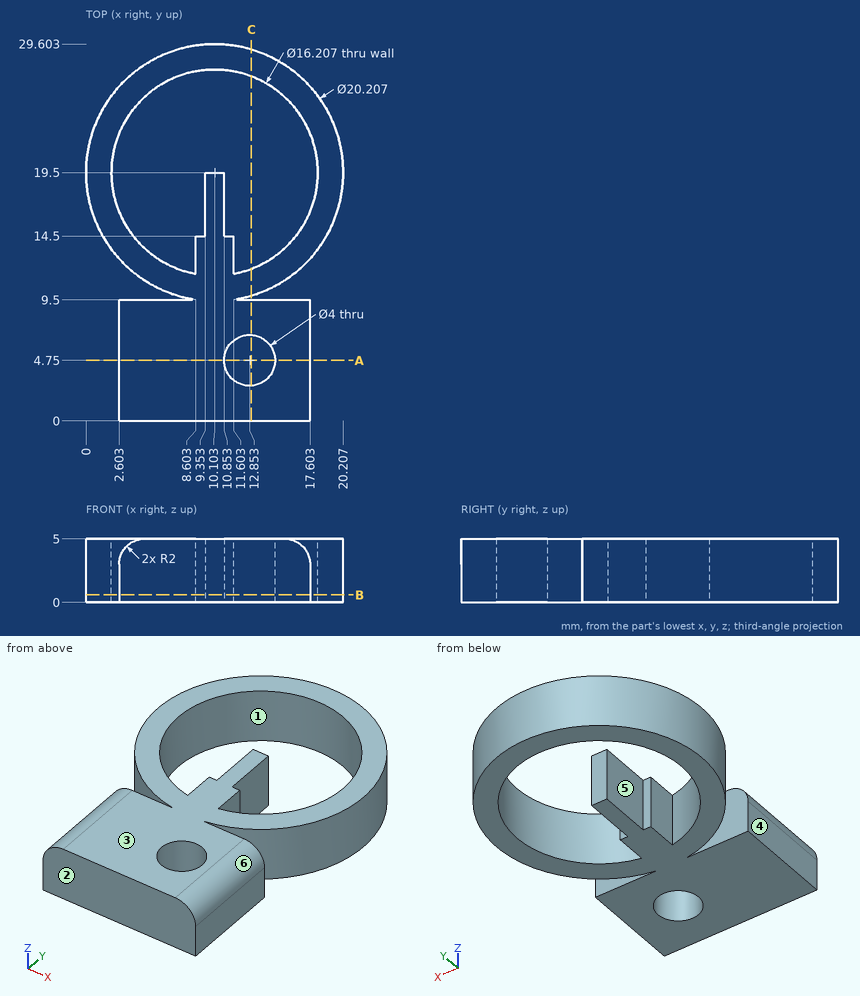
Input: dimensioned drawing with shaded views. Units: mm. Origin: part minimum x, y, z. A direction names the side the tool comes from. Round coordinates to 2 decimals unless told otherwise and drop trailing zeros. Order: outer loops, then holes, each group sorted by start corner. A loop starts at its lowest first (then second) coordinate and runs counter-clockwise, first axis right, second up. Notation, with made-up numbers: M 10,-8.75 L 65,-8.75 A32 cw 65,26.25 Z; hole C 6,7.5 d6. An arc over 180 degrees is marked long. Use one line per item in the form item = value. Start each with the question number.
Q1. Cut plane C-C (x = 13). Return loops of the section in (y, z) (1 decimal).
Q2. Cut plane A-A (y = 4.75). Return loops of the section in (x, z).
Q3. Access query for the marked faces 4, 5 and 6. Directions: +Z, -Z, +X, -X, +Y, -Y. A direction counts if a zero-diameter tool reaches every point of the face in a straight line with its end or side. Return the directions, or none.
Q4. Cut plane B-B (z = 0.6). Count the separate pieces of the cut face and the enclosed holes in it, and give its area (3 significant figures).
Q5. Mould query, pull axis Y, two halves, no side actions, for the marked faces 1, 2 and 3. Classes: +Y half, -Y half, draft (parallel to the pull), parting line (faces both ways), or undercut.
Q6. Pin query (flat end, axial travel): pin 1 Ø0.9 at (y, z) = (4.5, 1) entering from +X; pin 2 Ø2 at (x, z) = (3.5, 1.5) entering from +Y; pin 3 Ø2.5 at (x, z) = (14.5, 3) entering from +Y. Return the tip coordinate at first contact, or that it passes through.
Q7. Material intervals for line 1 (X direction, y = 19.25, z = 0.65); line 2 (Y direction, x = 16.75, z = 4.1) (1 decimal); line 3 (X direction, y = 18, z = 4.6) (1 decimal), sorted ascending. Write a range as [from, to].
Geometry results:
q1.outline = M 0,0 L 2.8,0 L 2.8,5 L 0,5 Z; M 6.7,0 L 9.5,0 L 9.5,5 L 6.7,5 Z; M 9.8,0 L 11.9,0 L 11.9,5 L 9.8,5 Z; M 27.1,0 L 29.2,0 L 29.2,5 L 27.1,5 Z
q2.outline = M 2.6,0 L 10.85,0 L 10.85,5 L 4.6,5 A2 ccw 2.6,3 Z; M 14.85,0 L 17.6,0 L 17.6,3 A2 ccw 15.6,5 L 14.85,5 Z
q3.face_4 = +Z, -Z, -X, -Y
q3.face_5 = +Z, -Z
q3.face_6 = +Z, +X, -Y
q4.separate_pieces = 1
q4.enclosed_holes = 2
q4.area = 261 mm^2
q5.face_1 = undercut
q5.face_2 = -Y half
q5.face_3 = draft
q6.pin_1 = 17.6
q6.pin_2 = 27.91
q6.pin_3 = 29.1
q7.line_1 = [0, 2], [9.35, 10.85], [18.2, 20.2]
q7.line_2 = [0, 9.5], [11.9, 14.9], [24.1, 27.1]
q7.line_3 = [0.1, 2.1], [9.4, 10.9], [18.1, 20.1]
